Read the model definition and answer for the solid it produces. Units are mm, in the model's axes. Face numbers are marked on the shaded views. A direction names the side the tool comes from. Give positions to 0.01 mm unless a question says otherwise; leave off trailing zeros. Order: outer loops, then holes, each group sorted by start corner. A loop starts at its lowest first (then second) coordinate and runs counter-clockwise, first axis right, second up. Notation, with made-up numbers: M 26.5,67 L 49.5,67 A9 cw 49.5,72 Z; hole C 15.5,51.5 d6. An arc over 180 degrees is marked long. One line per item, written item: value.
from build123d import *

# Parameters (mm, degrees)
F0_W     = 127
F0_H     = 76.2
F1_DEPTH = 63.5
F2_W     = 38.1
F2_H     = 50.8
F3_DEPTH = 50.8
F4_W     = 38.1
F4_H     = 50.8
F5_DEPTH = 50.8
F7_DEPTH = 76.201


with BuildPart() as f1:
    # F0 (on Front) → F1 (new body)
    with BuildSketch(Plane.XZ):
        with Locations((-31.45163, -18.051595)):
            Rectangle(F0_W, F0_H)
    extrude(amount=F1_DEPTH)

    # F2 (on face) → F3 (cut)
    with BuildSketch(Plane.YZ.offset(32.04837)):
        with Locations((-44.45, -5.351595)):
            Rectangle(F2_W, F2_H)
    extrude(amount=-F3_DEPTH, mode=Mode.SUBTRACT)

    # F4 (on face) → F5 (cut)
    with BuildSketch(Plane(origin=(-94.95163, 0, 0), x_dir=(0, -1, 0), z_dir=(-1, 0, 0))):
        with Locations((44.45, -5.351595)):
            Rectangle(F4_W, F4_H)
    extrude(amount=-F5_DEPTH, mode=Mode.SUBTRACT)

    # F6 (on face) → F7 (cut, through all)
    with BuildSketch(Plane(origin=(-44.15163, 0, 0), x_dir=(0, -1, 0), z_dir=(-1, 0, 0))):
        Polygon((63.5, 20.048405), (25.4, 20.048405), (63.5, -30.751595), align=None)
    extrude(amount=-F7_DEPTH, mode=Mode.SUBTRACT)


solid = f1.part
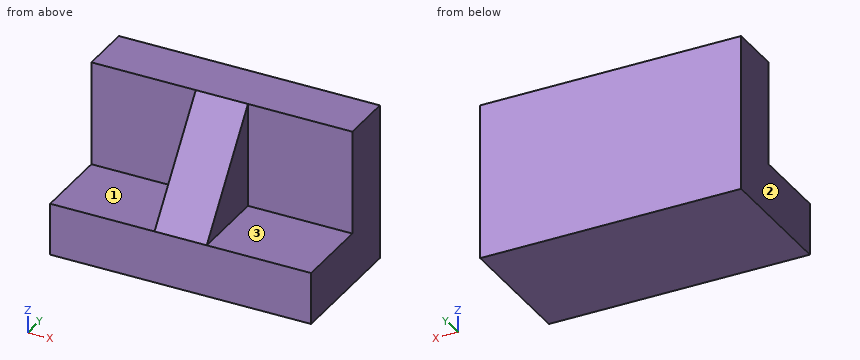
1) Find section D-D, the plane x = -58.5. Write down the section's boundary in (y, z), plus the area to 3 significant figures.
Reported:
outline: M -63.5,-56.15 L 0,-56.15 L 0,20.05 L -25.4,20.05 L -25.4,-30.75 L -63.5,-30.75 Z
area: 2,900 mm^2
2) Find section A-A, the plane x = -28.5. Write down the section's boundary in (y, z).
Reported:
outline: M -63.5,-56.15 L 0,-56.15 L 0,20.05 L -25.4,20.05 L -63.5,-30.75 Z
3) Find section B-B, the plane z = -19.5. Write down the section's boundary in (x, y), plus the area to 3 significant figures.
Reported:
outline: M -94.95,-25.4 L -44.15,-25.4 L -44.15,-55.06 L -18.75,-55.06 L -18.75,-25.4 L 32.05,-25.4 L 32.05,0 L -94.95,0 Z
area: 3,980 mm^2
4) Consider probe 1 along Y at (x, z) = (-13.5, 2.5); probe 2 along X at (y, z) = (-30, 0.5); probe 3 along Z at (x, y) = (-64.5, -50.5). Determine where each line is inside the solid, lowest interval first.
Reported:
probe 1: y = -25.4 to 0
probe 2: x = -44.15 to -18.75
probe 3: z = -56.15 to -30.75
5) Find section C-C, the plane y = -47. Write down the section's boundary in (x, z).
Reported:
outline: M -94.95,-56.15 L 32.05,-56.15 L 32.05,-30.75 L -18.75,-30.75 L -18.75,-8.75 L -44.15,-8.75 L -44.15,-30.75 L -94.95,-30.75 Z
6) Which of the six approach directions +Z, -Z, +X, -X, +Y, -Y give full straight-line access (tool end or side, diameter ignored) to the marked faces 1, 2 and 3?
Reported:
face 1: +Z, -X, -Y
face 2: +Z, -Z, -X, +Y, -Y
face 3: +Z, +X, -Y
7) Each of these flat-tipped pins is pushed along its axis until it touches: pin 1 Ø4 at (x, z) = (-6, -12.5) entering from -Y; pin 2 Ø10 at (x, z) = (-20.5, 4.5) entering from -Y; pin 3 Ø2 at (x, y) = (-32, -36) entering from +Z. Where does it stop, or does it pass through?
Reported:
pin 1: stops at y = -25.4
pin 2: stops at y = -40.81
pin 3: stops at z = 7.25
